Can you work these out from the model? Positions are in its coordinate system, mm. A direction names the side the tool comes from. Round coordinates to 2 decimals unless told otherwise and drop trailing zeros. Write each loop counter-clockwise with the first axis right and the second up, starting at its lowest first coordinate (ties: lowest second). Pieces come first, ordered by that corner, then holes. Notation, with made-up numbers: M 30,52.5 L 50,52.5 A23 ccw 50,70.5 Z; hole C -1,-31.75 d1. An arc over 180 degrees is marked long. Answer in a Markdown table with one row per item. Add a question column.
(1) Suppose I cut it at C-C, the plane z = 7.25. Write out the boundary of the cut face in (x, y).
(2) Suppose I cut it at A-A, the plane x = 0. Write out the boundary of the cut face in (y, z).
(3) For faces 5 (the face through (-0.59, 4.46, 4.94)), 6 (the face through (0, -5, 9)), 7 (the face through (14, 0, 1.5)), 8 (the face through (4, -4, 10)), 9 (the face through (-4.09, 3.13, 0.51)), which set-ups out of +Z, -Z, +X, -X, +Y, -Y let a thin tool reach every point of the face, with its end or its side?
(4) If I drill on probe 1 along Y at (x, z) = (0, 9.5); probe 2 along Z at (x, y) = (12, -7); probe 3 along X at (y, z) = (0, 7.75), over which ranges is the centre line in solid material (lowest first)?
(5) Suppose I cut it at D-D, the plane y = 8. Write out the boundary of the cut face in (x, z).
(6) If we mould it in two halves opening along Z, with no side actions, what happens to faces 1 (the face through (4, 4, 0)), 2 (the face through (14, 0, 8.5)), 3 (the face through (4.91, 1.55, 9.51)), 4 (the face through (-2.93, -13.18, 4.95))? For each: released by +Z, released by -Z, zero draft, split by the parting line, or undercut.
(7) I'm going to push flat-ended pins straight in: pin 1 (6 mm diameter, centred on x = -3, z = 6.5, fed in from +Y); pin 2 (8 mm diameter, centred on x = 0.5, y = 1, fed in from -Z); pin 3 (5 mm diameter, centred on y = -4, z = 7.5, fed in from -X). Where does each tip first touch, or does it pass through?
from build123d import *

# Parameters (mm, degrees)
SKETCH1_R           = 13.5
SKETCH1_R_2         = 4.5
BOSS_EXTRUDE1_DEPTH = 10
SKETCH2_R           = 5.15
CUT_EXTRUDE1_DEPTH  = 1
CUT_EXTRUDE2_START  = -1
SKETCH3_R           = 5.15
CUT_EXTRUDE2_DEPTH  = 1
BOSS_EXTRUDE2_START = -1.5
SKETCH4_R           = 16.5
SKETCH4_R_2         = 5.15
BOSS_EXTRUDE2_DEPTH = 1.5
SKETCH5_R           = 16.5
SKETCH5_R_2         = 5.15
BOSS_EXTRUDE3_DEPTH = 1.5


with BuildPart() as part:
    # Sketch1 → Boss-Extrude1 (new body)
    with BuildSketch(Plane.XY):
        Circle(SKETCH1_R)
        Circle(SKETCH1_R_2, mode=Mode.SUBTRACT)
    extrude(amount=BOSS_EXTRUDE1_DEPTH)

    # Sketch2 → Cut-Extrude1 (cut)
    with BuildSketch(Plane.XY.offset(10)):
        Circle(SKETCH2_R)
    extrude(amount=-CUT_EXTRUDE1_DEPTH, mode=Mode.SUBTRACT)

    # Sketch3 → Cut-Extrude2 (cut)
    with BuildSketch(Plane(origin=(0, 0, 0), x_dir=(-1, 0, 0), z_dir=(0, 0, -1)).offset(CUT_EXTRUDE2_START)):
        with Locations(Location((0, 0, 0), (0, 0, 180))):
            Circle(SKETCH3_R)
    extrude(amount=CUT_EXTRUDE2_DEPTH, mode=Mode.SUBTRACT)

    # Sketch4 → Boss-Extrude2 (add)
    with BuildSketch(Plane(origin=(0, 0, 0), x_dir=(-1, 0, 0), z_dir=(0, 0, -1)).offset(BOSS_EXTRUDE2_START)):
        Circle(SKETCH4_R)
        with Locations(Location((0, 0, 0), (0, 0, 180))):
            Circle(SKETCH4_R_2, mode=Mode.SUBTRACT)
    extrude(amount=BOSS_EXTRUDE2_DEPTH)

    # Sketch5 → Boss-Extrude3 (add)
    with BuildSketch(Plane.XY.offset(10)):
        with Locations(Location((0, 0, 0), (0, 0, 180))):
            Circle(SKETCH5_R)
        Circle(SKETCH5_R_2, mode=Mode.SUBTRACT)
    extrude(amount=-BOSS_EXTRUDE3_DEPTH)


solid = part.part
Calculated:
| question | item | result |
|---|---|---|
| 1 | outline | C 0,0 d27; hole C 0,0 d9 |
| 2 | outline | M -16.5,0 L -5.15,0 L -5.15,1 L -4.5,1 L -4.5,9 L -5.15,9 L -5.15,10 L -16.5,10 L -16.5,8.5 L -13.5,8.5 L -13.5,1.5 L -16.5,1.5 Z; M 4.5,1 L 5.15,1 L 5.15,0 L 16.5,0 L 16.5,1.5 L 13.5,1.5 L 13.5,8.5 L 16.5,8.5 L 16.5,10 L 5.15,10 L 5.15,9 L 4.5,9 Z |
| 3 | face 5 | +Z, -Z |
| 3 | face 6 | +Z |
| 3 | face 7 | none |
| 3 | face 8 | +Z, +X, -X, +Y, -Y |
| 3 | face 9 | -Z |
| 4 | probe 1 | -16.5 to -5.15, 5.15 to 16.5 |
| 4 | probe 2 | 0 to 1.5, 8.5 to 10 |
| 4 | probe 3 | -13.5 to -4.5, 4.5 to 13.5 |
| 5 | outline | M -14.43,0 L 14.43,0 L 14.43,1.5 L 10.87,1.5 L 10.87,8.5 L 14.43,8.5 L 14.43,10 L -14.43,10 L -14.43,8.5 L -10.87,8.5 L -10.87,1.5 L -14.43,1.5 Z |
| 6 | face 1 | released by -Z |
| 6 | face 2 | undercut |
| 6 | face 3 | zero draft |
| 6 | face 4 | undercut |
| 7 | pin 1 | y = 16.48 |
| 7 | pin 2 | z = 1 |
| 7 | pin 3 | x = -16.41 |
